Work out the finished part from the listing and answer in its coordinate system (mm). Face numbers are marked on the shaded views. Coordinates: 2 decimals unless noted, no trailing zeros. Loops run counter-clockwise (first coordinate to the right, second up) from the corner with the lowest first, then second, coordinate; pieces in that order, holes last. Notation, with made-up numbers: (62, 65) - (105, 65) arc R16 cw to (105, 84) - close; hole circle Ø11 at (-15, 26.25). An arc over 180 degrees is marked (long way). Write each question's results on one line, items separated by ' | '. Start each with the question number.
1. A cutting plane is placed at A-A on x = 0. Determine the outline of the cut face in (y, z), then the cut area to 3 significant figures.
2. Determine the mould class of the marked faces 1, 2 and 3 for opening direction Z: released by +Z, released by -Z, zero draft, split by the parting line, or undercut.
3. A cutting plane is placed at C-C on y = -0.4. Determine the outline of the cut face in (x, z), then the cut area to 3 significant figures.
4. Find the intervals of material crossed by line 1 along X through (y, z) = (0.1, 0); line 2 along Z through (x, y) = (0, -0.6); line 3 along X through (y, z) = (0.9, 0.6), in increasing order. Write a range as [from, to].
5. A cutting plane is placed at B-B on z = 0. Determine the outline of the cut face in (x, y), then the cut area to 3 significant figures.
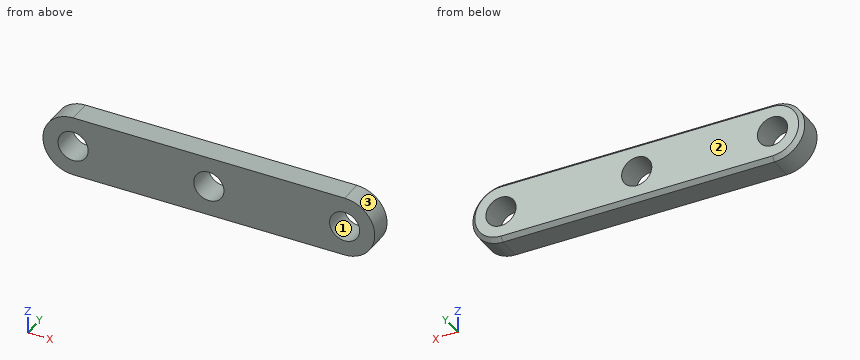
from build123d import *

# Parameters (mm, degrees)
SKETCH1_R           = 1.5
BOSS_EXTRUDE1_DEPTH = 1.35
CHAMFER1_SIZE       = 0.4


with BuildPart() as part:
    # Sketch1 → Boss-Extrude1 (new body, symmetric)
    with BuildSketch(Plane(origin=(0, 0, 0), x_dir=(1, 0, 0), z_dir=(0, 1, 0))):
        with BuildLine():
            Line((-13.5, 3), (13.5, 3))
            ThreePointArc((13.5, 3), (16.5, 0), (13.5, -3))
            Line((13.5, -3), (-13.5, -3))
            ThreePointArc((-13.5, -3), (-16.5, 0), (-13.5, 3))
        make_face()
        with Locations((-13.5, 0)):
            Circle(SKETCH1_R, mode=Mode.SUBTRACT)
        with Locations((13.5, 0)):
            Circle(SKETCH1_R, mode=Mode.SUBTRACT)
        Circle(SKETCH1_R, mode=Mode.SUBTRACT)
    extrude(amount=BOSS_EXTRUDE1_DEPTH, both=True)

    # Chamfer1
    chamfer1_edges = [part.edges().sort_by_distance(p)[0] for p in [
        (16.5, 1.35, 0),
        (0, 1.35, -3),
        (-16.5, 1.35, 0),
        (0, 1.35, 3),
    ]]
    chamfer(chamfer1_edges, length=CHAMFER1_SIZE)


solid = part.part
Values:
1) outline: (-1.35, -3) - (0.95, -3) - (1.35, -2.6) - (1.35, -1.5) - (-1.35, -1.5) - close; (-1.35, 1.5) - (1.35, 1.5) - (1.35, 2.6) - (0.95, 3) - (-1.35, 3) - close | area: 7.94 mm^2
2) face 1: undercut | face 2: zero draft | face 3: split by the parting line
3) outline: (-13.5, -3) - (13.5, -3) arc R3 ccw to (13.5, 3) - (-13.5, 3) arc R3 ccw to start; hole circle Ø3 at (-13.5, 0); hole circle Ø3 at (0, 0); hole circle Ø3 at (13.5, 0) | area: 169 mm^2
4) line 1: [-16.5, -15], [-12, -1.5], [1.5, 12], [15, 16.5] | line 2: [-3, -1.5], [1.5, 3] | line 3: [-16.44, -14.87], [-12.13, -1.37], [1.37, 12.13], [14.87, 16.44]
5) outline: (-16.5, -1.35) - (-15, -1.35) - (-15, 1.35) - (-16.1, 1.35) - (-16.5, 0.95) - close; (-12, -1.35) - (-1.5, -1.35) - (-1.5, 1.35) - (-12, 1.35) - close; (1.5, -1.35) - (12, -1.35) - (12, 1.35) - (1.5, 1.35) - close; (15, -1.35) - (16.5, -1.35) - (16.5, 0.95) - (16.1, 1.35) - (15, 1.35) - close | area: 64.6 mm^2
